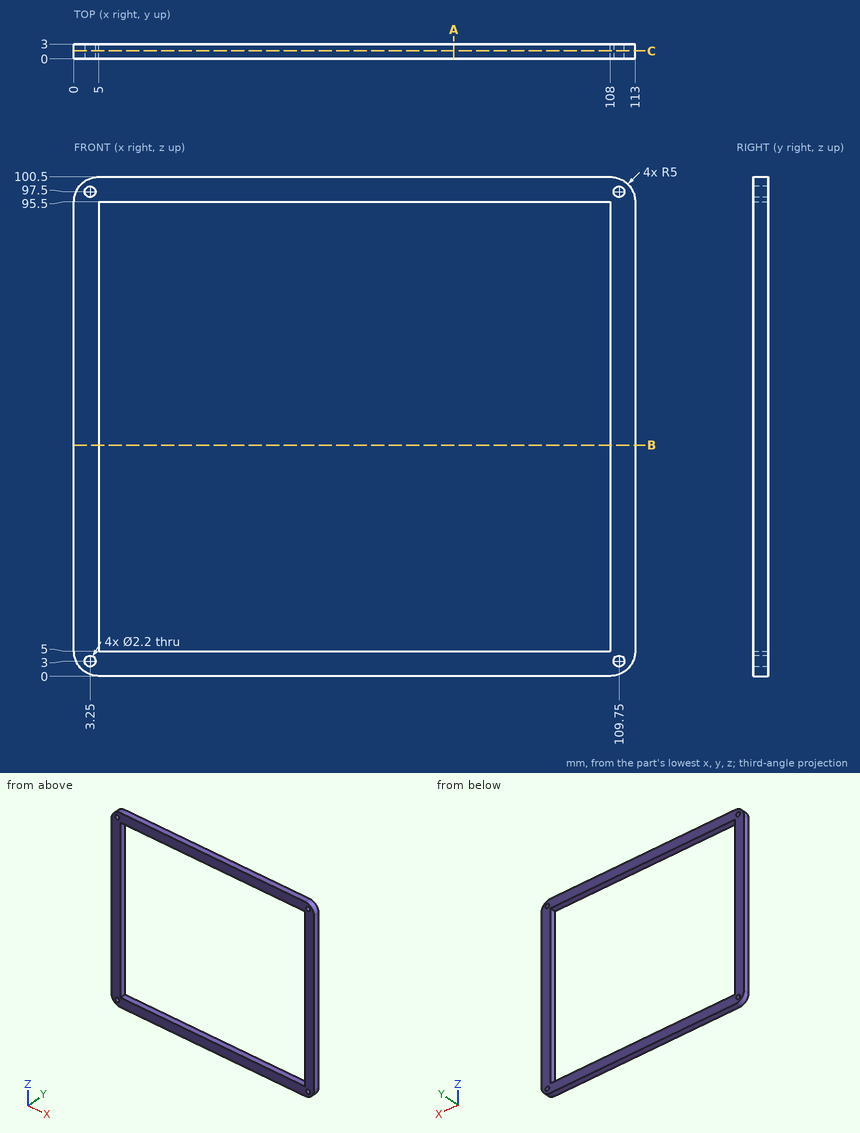
Geometry: see drawing. Coordinates: mm, zero at the bounding-box minimum. Coordinates: 2 decimals unless noted, no trailing zeros. Order: outer loops, then holes, each group sorted by start corner. A loop starts at its lowest first (then second) coordinate and runs counter-clockwise, first axis right, second up. Notation, with made-up numbers: M 72,13.5 L 117,13.5 A14 ccw 117,32.5 Z; hole C 73.5,72.5 d6. An arc over 180 degrees is marked long. Answer in a Markdown table with one row per item. Add a question column.
Q1. Line query: L1, parallel to X at y = 2.2, z = 88.5; L2, parallel to Z at x = 109.75, y = 1.7; L3, parallel to Z at x = 82, y = 2.55. Output: solid intervals per line, ascending.
Q2. Section query A-A on x = 76.5. Return the cut outline in (y, z), and give its area (3 significant figures).
Q3. Section query C-C on y = 1.6. Return the cut outline in (x, z), and give its area (3 significant figures).
Q4. Section query B-B on z = 46.5. Return the cut outline in (x, y).
Completed:
| question | item | result |
|---|---|---|
| 1 | L1 | x = 0 to 5, 108 to 113 |
| 1 | L2 | z = 0.32 to 1.9, 4.1 to 96.4, 98.6 to 100.18 |
| 1 | L3 | z = 0 to 5, 95.5 to 100.5 |
| 2 | outline | M 0,0 L 3,0 L 3,5 L 0,5 Z; M 0,95.5 L 3,95.5 L 3,100.5 L 0,100.5 Z |
| 2 | area | 30.0 mm2 |
| 3 | outline | M 0,5 A5 ccw 5,0 L 108,0 A5 ccw 113,5 L 113,95.5 A5 ccw 108,100.5 L 5,100.5 A5 ccw 0,95.5 Z; hole C 3.25,3 d2.2; hole C 3.25,97.5 d2.2; hole M 5,5 L 108,5 L 108,95.5 L 5,95.5 Z; hole C 109.75,3 d2.2; hole C 109.75,97.5 d2.2 |
| 3 | area | 2,000 mm2 |
| 4 | outline | M 0,0 L 5,0 L 5,3 L 0,3 Z; M 108,0 L 113,0 L 113,3 L 108,3 Z |
